Geometry check sheet. Reference: the model listing, model coordinates, mm. A direction names the side the tool comes from. Round coordinates to 2 decimals unless told otherwise and drop trailing zeros. Write each loop counter-clockwise with the first axis right and the second up, starting at its lowest first coordinate (ties: lowest second). Pieces come first, ordered by that corner, then holes. Notation, with made-up numbers: M -17,-21 L 40,-21 A26 ccw 40,-7 Z; hole C 32.25,6 d5. An arc over 180 degrees is marked long. Use a Markdown table: item, result.
```python
from build123d import *

# Parameters (mm, degrees)
SKETCH1_R            = 15.5
SKETCH1_R_2          = 12.5
BOSS_EXTRUDE1_DEPTH  = 0.4
SKETCH2_R            = 15.5
SKETCH2_R_2          = 4.5
BOSS_EXTRUDE2_DEPTH  = 4.8
M4_CLEARANCE_HOLE1_D = 4.3


with BuildPart() as part:
    # Sketch1 → Boss-Extrude1 (new body)
    with BuildSketch(Plane.XY):
        Circle(SKETCH1_R)
        Circle(SKETCH1_R_2, mode=Mode.SUBTRACT)
    extrude(amount=BOSS_EXTRUDE1_DEPTH)

    # Sketch2 → Boss-Extrude2 (add)
    with BuildSketch(Plane(origin=(0, 0, 0), x_dir=(-1, 0, 0), z_dir=(0, 0, -1))):
        Circle(SKETCH2_R)
        Circle(SKETCH2_R_2, mode=Mode.SUBTRACT)
    extrude(amount=BOSS_EXTRUDE2_DEPTH)

    # M4 Clearance Hole1 (through all)
    with Locations(Plane(origin=(0, 0, -4.8), x_dir=(-1, 0, 0), z_dir=(0, 0, -1))):
        with Locations((0, 8.5), (7.361215932, -4.25), (-7.361215932, -4.25)):
            Hole(M4_CLEARANCE_HOLE1_D / 2)


solid = part.part
```
Item 1: Cross-section at C-C, the plane z = -3.85. Record the cut outline in (x, y).
Outcome:
| item | result |
|---|---|
| outline | C 0,0 d31; hole C -7.36,-4.25 d4.3; hole C 0,0 d9; hole C 0,8.5 d4.3; hole C 7.36,-4.25 d4.3 |
Item 2: Cross-section at B-B, the plane x = 0. Record the cut outline in (y, z), and give its area (3 significant figures).
Outcome:
| item | result |
|---|---|
| outline | M -15.5,-4.8 L -4.5,-4.8 L -4.5,0 L -12.5,0 L -12.5,0.4 L -15.5,0.4 Z; M 4.5,-4.8 L 6.35,-4.8 L 6.35,0 L 4.5,0 Z; M 10.65,-4.8 L 15.5,-4.8 L 15.5,0.4 L 12.5,0.4 L 12.5,0 L 10.65,0 Z |
| area | 87.4 mm2 |
Item 3: Access from +Z, -Z, +X, -X, +Y, -Y to the whole of each face (thin tool, end or side, straight path). Record for faces 3 (the face through (5.655, -5.558, -2.366)), 4 (the face through (11.923, 3.755, 0.197)).
Outcome:
| item | result |
|---|---|
| face 3 | +Z, -Z |
| face 4 | +Z |
Item 4: Material ranges on line 1 along Y through (x, z) = (0, 0.3); line 2 along Y through (x, z) = (0, -3.75); line 3 along X through (y, z) = (-3, -0.75), recorded low to high. Write a range as from..to.
Outcome:
| item | result |
|---|---|
| line 1 | y = -15.5..-12.5, 12.5..15.5 |
| line 2 | y = -15.5..-4.5, 4.5..6.35, 10.65..15.5 |
| line 3 | x = -15.21..-9.11, -5.61..-3.35, 3.35..5.61, 9.11..15.21 |
Item 5: Cross-section at A-A, the plane y = 0. Record the cut outline in (x, z).
Outcome:
| item | result |
|---|---|
| outline | M -15.5,-4.8 L -4.5,-4.8 L -4.5,0 L -12.5,0 L -12.5,0.4 L -15.5,0.4 Z; M 4.5,-4.8 L 15.5,-4.8 L 15.5,0.4 L 12.5,0.4 L 12.5,0 L 4.5,0 Z |
Item 6: Go/stop test with flat-tipped pins: pin 1 (12.5 mm diameter, centred on x = 2, y = -5, fed in from +Z); pin 2 (1.5 mm diameter, centred on y = 1.5, z = -2, fed in from +X); pin 3 (1.5 mm diameter, centred on x = -8, z = -0.5, fed in from +Y). Record where each tip stops, or that it passes through.
Outcome:
| item | result |
|---|---|
| pin 1 | stops at z = 0 |
| pin 2 | stops at x = 15.48 |
| pin 3 | stops at y = 13.7 |
Item 7: Cross-section at D-D, the plane y = -5.5. Record the cut outline in (x, z).
Outcome:
| item | result |
|---|---|
| outline | M -14.49,-4.8 L -9.11,-4.8 L -9.11,0 L -11.22,0 L -11.22,0.4 L -14.49,0.4 Z; M -5.61,-4.8 L 5.61,-4.8 L 5.61,0 L -5.61,0 Z; M 9.11,-4.8 L 14.49,-4.8 L 14.49,0.4 L 11.22,0.4 L 11.22,0 L 9.11,0 Z |
Item 8: Mould release check, pull along Y, two halves, no side actions. Record for faces 1 (the face through (-0.28, 10.63, -2.37)), 2 (the face through (1, 13, 0.4)): +Y half, -Y half, draft (parallel to the pull), parting line (faces both ways), or undercut.
Outcome:
| item | result |
|---|---|
| face 1 | undercut |
| face 2 | draft |
